Part model, mm, in its own coordinate system. Face numbers are marked on the shaded views. A direction names the side the tool comes from. Give positions to 0.01 mm unless a question says otherwise; leave off trailing zeros. Order: outer loops, then holes, each group sorted by start corner. A loop starts at its lowest first (then second) coordinate and runs counter-clockwise, first axis right, second up. Notation, with made-up numbers: (52.25, 56) -> (85.25, 56) arc R15 cw to (85.25, 72) -> close; hole circle Ø10 at (43.5, 17). An arc over 180 degrees is marked (long way). Write item = value, one per line. Start each with the question number.
Item 1: Drill centre lines: line 1 along X through (y, z) = (3.5, 4.5); line 2 along X through (y, z) = (5.75, -5.75); line 3 along X through (y, z) = (3.45, 0). Where is each one in solid material? Low to high.
Item 2: Pull direction X, two halves, no side cores. Call the marked faces 1, 2, 3 and 4: +X half, -X half, draft (parallel to the pull), parting line (faces both ways), or undercut.
Item 3: Band-saw the part on A-A on x = -1.5. Write the cut outline in (y, z).
Item 4: Band-saw the part on B-B on x = -38. Write the cut outline in (y, z).
Item 5: Flat gauge pins, fed straight in: P1, Ø2, axis at x = 38, y = 9, coming from the -Z side; P2, Ø6, axis at y = 5.5, z = 9, coming from the -X side; P3, Ø12.5, axis at x = -1, z = 3, coming from the +Y side. Where does each tip first touch, or does it go through?
Item 6: Band-saw the part on C-C on x = -15.5. Write the cut outline in (y, z), plus the area to 3 significant figures.
Item 7: Tool access for the marked faces 5, 6, 7 and 8: list every direction of +Z, -Z, +X, -X, +Y, -Y with a clear straight run to the whole face (end or side of a thin tool).
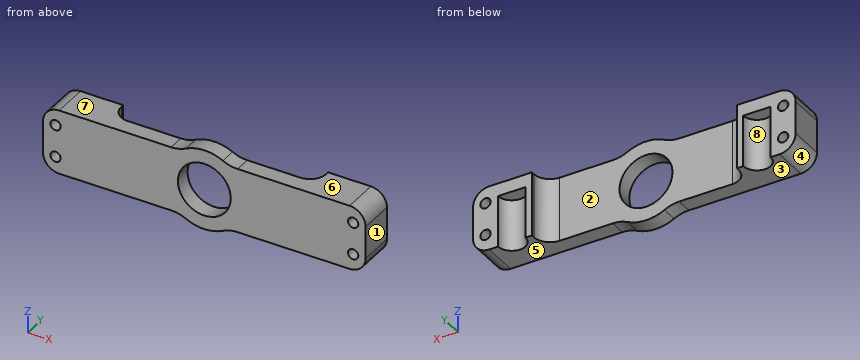
```python
from build123d import *

# Parameters (mm, degrees)
SKETCH1_W               = 88
SKETCH1_H               = 20
BOSS_EXTRUDE1_DEPTH     = 22
SKETCH2_R               = 4.25
CUT_EXTRUDE1_DEPTH      = 21
SKETCH7_R               = 12.5
BOSS_EXTRUDE2_DEPTH     = 22
SKETCH4_R               = 8.2
CUT_EXTRUDE3_DEPTH      = 23
FILLET2_R               = 10
SKETCH9_W               = 27
SKETCH9_H               = 11
CUT_EXTRUDE4_DEPTH      = 89
SKETCH10_W              = 63.5
SKETCH10_H              = 8
CUT_EXTRUDE5_DEPTH      = 13.5
CUT_EXTRUDE5_DEPTH_BACK = 13.5
FILLET3_R               = 5
SKETCH11_W              = 20
SKETCH11_H              = 11
BOSS_EXTRUDE3_DEPTH     = 6
SKETCH12_R              = 1.6
CUT_EXTRUDE6_DEPTH      = 12
FILLET4_R               = 5
BOSS_EXTRUDE4_DEPTH     = 4


with BuildPart() as part:
    # Sketch1 → Boss-Extrude1 (new body)
    with BuildSketch(Plane(origin=(0, 0, 0), x_dir=(1, 0, 0), z_dir=(0, 1, 0))):
        Rectangle(SKETCH1_W, SKETCH1_H)
    extrude(amount=BOSS_EXTRUDE1_DEPTH)

    # Sketch2 → Cut-Extrude1 (cut, through all)
    with BuildSketch(Plane.XY.offset(10)):
        with Locations((-38, 11)):
            Circle(SKETCH2_R)
        with Locations((38, 11)):
            Circle(SKETCH2_R)
    extrude(amount=-CUT_EXTRUDE1_DEPTH, mode=Mode.SUBTRACT)

    # Sketch7 → Boss-Extrude2 (add)
    with BuildSketch(Plane(origin=(0, 22, 0), x_dir=(1, 0, 0), z_dir=(0, 1, 0))):
        Circle(SKETCH7_R)
    extrude(amount=-BOSS_EXTRUDE2_DEPTH)

    # Sketch4 → Cut-Extrude3 (cut, through all)
    with BuildSketch(Plane(origin=(0, 22, 0), x_dir=(1, 0, 0), z_dir=(0, 1, 0))):
        Circle(SKETCH4_R)
    extrude(amount=-CUT_EXTRUDE3_DEPTH, mode=Mode.SUBTRACT)

    # Fillet2
    fillet2_edges = [part.edges().sort_by_distance(p)[0] for p in [
        (7.5, 11, -10),
        (7.5, 11, 10),
        (-7.5, 11, -10),
        (-7.5, 11, 10),
    ]]
    fillet(fillet2_edges, radius=FILLET2_R)

    # Sketch9 → Cut-Extrude4 (cut, through all)
    with BuildSketch(Plane.ZY.offset(44)):
        with Locations((0, 16.5)):
            Rectangle(SKETCH9_W, SKETCH9_H)
    extrude(amount=-CUT_EXTRUDE4_DEPTH, mode=Mode.SUBTRACT)

    # Sketch10 → Cut-Extrude5 (cut, two sides)
    with BuildSketch(Plane.XY) as cut_extrude5_sk:
        with Locations((0, 9)):
            Rectangle(SKETCH10_W, SKETCH10_H)
    extrude(amount=CUT_EXTRUDE5_DEPTH, mode=Mode.SUBTRACT)
    extrude(cut_extrude5_sk.sketch, amount=-CUT_EXTRUDE5_DEPTH_BACK, mode=Mode.SUBTRACT)

    # Fillet3
    fillet3_edges = [part.edges().sort_by_distance(p)[0] for p in [
        (31.75, 5, 0),
        (-31.75, 5, 0),
    ]]
    fillet(fillet3_edges, radius=FILLET3_R)

    # Sketch11 → Boss-Extrude3 (add)
    with BuildSketch(Plane(origin=(44, 0, 0), x_dir=(0, 0, -1), z_dir=(1, 0, 0))):
        with Locations((0, 5.5)):
            Rectangle(SKETCH11_W, SKETCH11_H)
    boss_extrude3 = extrude(amount=BOSS_EXTRUDE3_DEPTH)

    # Sketch12 → Cut-Extrude6 (cut, through all)
    with BuildSketch(Plane(origin=(0, 11, 0), x_dir=(1, 0, 0), z_dir=(0, 1, 0))):
        with Locations((46.125, -5)):
            Circle(SKETCH12_R)
        with Locations((46.125, 5)):
            Circle(SKETCH12_R)
    cut_extrude6 = extrude(amount=-CUT_EXTRUDE6_DEPTH, mode=Mode.SUBTRACT)

    # Mirror1: Boss-Extrude3, Cut-Extrude6 across plane
    add(boss_extrude3.mirror(Plane(origin=(0, 0, 0), x_dir=(0, 0, 1), z_dir=(1, 0, 0))))
    add(cut_extrude6.mirror(Plane(origin=(0, 0, 0), x_dir=(0, 0, 1), z_dir=(1, 0, 0))), mode=Mode.SUBTRACT)

    # Fillet4
    fillet4_edges = [part.edges().sort_by_distance(p)[0] for p in [
        (50, 5.5, -10),
        (50, 5.5, 10),
        (-50, 5.5, 10),
        (-50, 5.5, -10),
    ]]
    fillet(fillet4_edges, radius=FILLET4_R)

    # Sketch13 → Boss-Extrude4 (add)
    with BuildSketch(Plane.XY.offset(10)):
        with BuildLine():
            Line((-42.25, 11), (-33.75, 11))
            ThreePointArc((-33.75, 11), (-38, 6.75), (-42.25, 11))
        make_face()
        with BuildLine():
            Line((33.75, 11), (42.25, 11))
            ThreePointArc((42.25, 11), (38, 6.75), (33.75, 11))
        make_face()
    extrude(amount=-BOSS_EXTRUDE4_DEPTH)


solid = part.part
```
Values found:
q1.line_1 = -50 to -47.64, -44.61 to -6.85, 6.85 to 44.61, 47.64 to 50
q1.line_2 = -49.94 to -47.54, -44.71 to -29.38, 29.38 to 44.71, 47.54 to 49.94
q1.line_3 = -50 to -8.2, 8.2 to 50
q2.face_1 = +X half
q2.face_2 = undercut
q2.face_3 = draft
q2.face_4 = -X half
q3.outline = (0, -12.41) -> (5, -12.41) -> (5, -8.06) -> (0, -8.06) -> close; (0, 8.06) -> (5, 8.06) -> (5, 12.41) -> (0, 12.41) -> close
q4.outline = (0, -10) -> (6.75, -10) -> (6.75, 6) -> (11, 6) -> (11, 10) -> (0, 10) -> close
q5.P1 = 6
q5.P2 = -49.9
q5.P3 = 5
q6.outline = (0, -10) -> (5, -10) -> (5, 10) -> (0, 10) -> close
q6.area = 100 mm^2
q7.face_5 = -Z, +X, +Y, -Y
q7.face_6 = +Z, +X, +Y, -Y
q7.face_7 = +Z, -X, +Y, -Y
q7.face_8 = -Z, +Y
